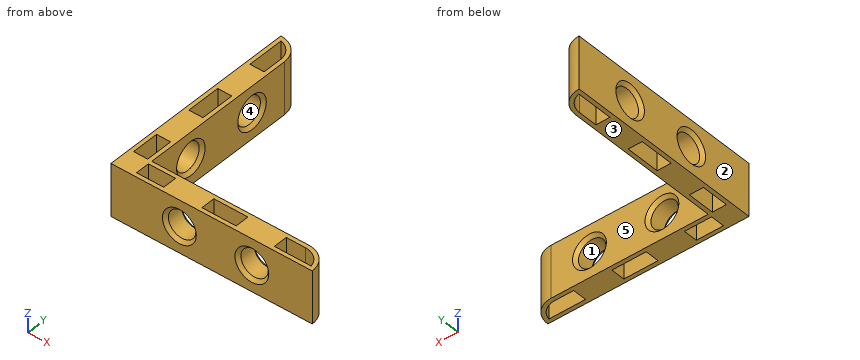
```python
from build123d import *

# Parameters (mm, degrees)
EXTRUDE_1_DEPTH            = 6.5
EXTRUDE_START              = -6.5
SKETCH_2_W                 = 5.5
SKETCH_2_H                 = 5.5
SKETCH_2_H_2               = 9.5
SKETCH_2_W_2               = 9.5
EXTRUDE_2_DEPTH            = 13
EXTRUDE_3_DEPTH            = 1
HOLE_WIZARD_M81_AT_2_COUNT = 2
HOLE_WIZARD_M81_AT_2_PITCH = 18


with BuildPart() as part:
    # Эскиз1 → Бобышка-Вытянуть1 (new body, symmetric)
    with BuildSketch(Plane.XY):
        with BuildLine():
            Line((0, 50), (0, 0))
            Line((0, 0), (50, 0))
            ThreePointArc((50, 0), (48.389087297, 3.889087297), (44.5, 5.5))
            Line((44.5, 5.5), (5.5, 5.5))
            Line((5.5, 5.5), (5.5, 44.5))
            ThreePointArc((5.5, 44.5), (3.889087297, 48.389087297), (0, 50))
        make_face()
        with BuildLine():
            Line((1, 48.887482194), (1, 1))
            Line((1, 1), (48.887482194, 1))
            ThreePointArc((48.887482194, 1), (47.30624304, 3.51781182), (44.5, 4.5))
            Line((44.5, 4.5), (4.5, 4.5))
            Line((4.5, 4.5), (4.5, 44.5))
            ThreePointArc((4.5, 44.5), (3.51781182, 47.30624304), (1, 48.887482194))
        make_face(mode=Mode.SUBTRACT)
    extrude(amount=EXTRUDE_1_DEPTH, both=True)

    # Эскиз2 → Бобышка-Вытянуть2 (add)
    with BuildSketch(Plane.XY.offset(EXTRUDE_START)):
        with Locations((2.75, 2.75)):
            Rectangle(SKETCH_2_W, SKETCH_2_H)
        with Locations((2.75, 35)):
            Rectangle(SKETCH_2_W, SKETCH_2_H_2)
        with Locations((2.75, 17)):
            Rectangle(SKETCH_2_W, SKETCH_2_H_2)
        with Locations((17, 2.75)):
            Rectangle(SKETCH_2_W_2, SKETCH_2_H)
        with Locations((35, 2.75)):
            Rectangle(SKETCH_2_W_2, SKETCH_2_H)
    extrude(amount=EXTRUDE_2_DEPTH)

    # Эскиз3 → Бобышка-Вытянуть3 (add, symmetric)
    with BuildSketch(Plane.XY):
        with BuildLine():
            Line((0, 0), (50, 0))
            ThreePointArc((50, 0), (48.389087297, 3.889087297), (44.5, 5.5))
            Line((44.5, 5.5), (5.5, 5.5))
            Line((5.5, 5.5), (5.5, 44.5))
            ThreePointArc((5.5, 44.5), (3.889087297, 48.389087297), (0, 50))
            Line((0, 50), (0, 0))
        make_face()
    extrude(amount=EXTRUDE_3_DEPTH, both=True)

    # Эскиз5 → Отверстие обработанное метчиком M81 (revolve, cut)
    with BuildSketch(Plane.ZX.offset(35)):
        Polygon((0, 0), (0, 5.5), (4.2, 5.5), (3.4, 4.7), (3.4, 0.8), (4.2, 0), align=None)
    hole_wizard_m81 = revolve(axis=Axis((-6.35, 35, 0), (1, 0, 0)), mode=Mode.SUBTRACT)

    # Отверстие обработанное метчиком M81 at 2: Отверстие обработанное метчиком M81 ×2
    with Locations(*[(0, -i * HOLE_WIZARD_M81_AT_2_PITCH, 0) for i in range(1, HOLE_WIZARD_M81_AT_2_COUNT)]):
        add(hole_wizard_m81, mode=Mode.SUBTRACT)

    # Зеркальное отражение1: Отверстие обработанное метчиком M81 across plane
    add(hole_wizard_m81.mirror(Plane(origin=(0, 0, 0), x_dir=(0, 0, 1), z_dir=(-0.707106781, 0.707106781, 0))), mode=Mode.SUBTRACT)

    # Зеркальное отражение1 copy 1 sketch → Зеркальное отражение1 copy 1 (revolve, cut)
    with BuildSketch(Plane(origin=(17, 0, 0), x_dir=(0, 0, 1), z_dir=(1, 0, 0))):
        Polygon((0, 0), (0, -5.5), (4.2, -5.5), (3.4, -4.7), (3.4, -0.8), (4.2, 0), align=None)
    revolve(axis=Axis((17, -6.35, 0), (0, -1, 0)), mode=Mode.SUBTRACT)


solid = part.part
```
Source: CAD feature listing. Evaluate the final solid. Frame: model axes, mm. Face numbers are marked on the shaded views. A direction names the side the tool comes from. Round coordinates to 2 decimals unless told otherwise and drop trailing zeros. Loops run counter-clockwise (first coordinate to the right, second up) from the corner with the lowest first, then second, coordinate; pieces in that order, holes last.
(1) Section query A-A (x = 35). Output: boundary loops of the cut face in (y, z).
From the geometry:
outline: (0, -6.5) - (5.5, -6.5) - (5.5, -4.2) - (4.7, -3.4) - (0.8, -3.4) - (0, -4.2) - close; (0, 4.2) - (0.8, 3.4) - (4.7, 3.4) - (5.5, 4.2) - (5.5, 6.5) - (0, 6.5) - close
(2) Access query for the marked faces 4 and 5. Directions: +Z, -Z, +X, -X, +Y, -Y. A direction counts if a zero-diameter tool reaches every point of the face in a straight line with its end or side. Return the directions, or none.
From the geometry:
face 4: +X, -X
face 5: +Z, -Z, +X, +Y
(3) Contact query for flat-ended pins moving along their axis: pin 1 Ø1.8 at (x, y) = (27.5, 3.5) entering from +Z; pin 2 Ø1.8 at (x, y) = (2, 44) entering from -Z; pin 3 Ø3 at (y, z) = (7.5, 3) entering from +X; pin 4 Ø3 at (y, z) = (25, -4) entering from -X. Output: stop coordinate, or through.
From the geometry:
pin 1: stops at z = 1
pin 2: stops at z = -1
pin 3: stops at x = 5.5
pin 4: stops at x = 0
(4) Section query D-D (z = 0). Give the number of separate pieces and of enclosed holes in the cut face, and give its area (3 significant figures).
From the geometry:
separate pieces: 5
enclosed holes: 0
area: 352 mm2
(5) Material intervals for probe 1 along Z at (x, y) = (2.5, 35); probe 2 along X at (y, z) = (10, 6); probe 3 along X at (y, z) = (2.7, 0), sorted ascending.
From the geometry:
probe 1: z = -6.5 to -3.4, 3.4 to 6.5
probe 2: x = 0 to 1, 4.5 to 5.5
probe 3: x = 0 to 13.6, 20.4 to 31.6, 38.4 to 49.29
(6) Pull-direction query (Z, two-part tool) for the marked faces 1, 2 and 3; classes: +Z half, -Z half, draft (parallel to the pull), parting line (faces both ways), or undercut.
From the geometry:
face 1: undercut
face 2: draft
face 3: -Z half
(7) Section query C-C (x = 10). Output: boundary loops of the cut face in (y, z).
From the geometry:
outline: (0, -6.5) - (1, -6.5) - (1, -1) - (4.5, -1) - (4.5, -6.5) - (5.5, -6.5) - (5.5, 6.5) - (4.5, 6.5) - (4.5, 1) - (1, 1) - (1, 6.5) - (0, 6.5) - close
